Model file for the job. Use its own axes, mm. A direction names the side the tool comes from. Coordinates: 2 decimals unless noted, no trailing zeros. Loops run counter-clockwise (first coordinate to the right, second up) from the corner with the lowest first, then second, coordinate; pieces in that order, holes last. Notation, with made-up numbers: M -37.5,66 L 0.5,66 A3 ccw 0.5,71 Z; hole C 31.5,17 d7. An arc over 180 degrees is marked long. One line per question, with ' | ' between items. Start each with the question number.
```python
from build123d import *

# Parameters (mm, degrees)
SKETCH_1_W      = 190
SKETCH_1_H      = 164
EXTRUDE_2_DEPTH = 105
SKETCH_1_5_W    = 95
SKETCH_1_5_H    = 204
EXTRUDE_3_DEPTH = 105
SKETCH_2_R      = 39.7
EXTRUDE_4_DEPTH = 55
SKETCH_3_R      = 39.7
EXTRUDE_5_DEPTH = 45
EXTRUDE_START   = 55
SKETCH_4_R      = 39.7
EXTRUDE_6_DEPTH = 55
EXTRUDE_START_2 = 45
SKETCH_5_R      = 39.7
EXTRUDE_7_DEPTH = 45


with BuildPart() as part:
    # Sketch 1 → Extrude 2 (new body)
    with BuildSketch(Plane(origin=(0, 0, 0), x_dir=(1, 0, 0), z_dir=(0, 1, 0))):
        Rectangle(SKETCH_1_W, SKETCH_1_H)
    extrude(amount=EXTRUDE_2_DEPTH)

    # Sketch 1_5 → Extrude 3 (add)
    with BuildSketch(Plane(origin=(0, 0, 0), x_dir=(1, 0, 0), z_dir=(0, 1, 0))):
        with Locations((-47.5, 0)):
            Rectangle(SKETCH_1_5_W, SKETCH_1_5_H)
    extrude(amount=EXTRUDE_3_DEPTH)

    # Sketch 2 → Extrude 4 (add)
    with BuildSketch(Plane.XY.offset(102)):
        with Locations((-47.5, 52.5)):
            Circle(SKETCH_2_R)
    extrude(amount=EXTRUDE_4_DEPTH)

    # Sketch 3 → Extrude 5 (add)
    with BuildSketch(Plane.XY.offset(82)):
        with Locations(Location((47.5, 52.5, 0), (0, 0, 180))):
            Circle(SKETCH_3_R)
    extrude(amount=EXTRUDE_5_DEPTH)

    # Sketch 4 → Extrude 6 (add)
    with BuildSketch(Plane(origin=(0, 0, -102), x_dir=(-1, 0, 0), z_dir=(0, 0, -1)).offset(EXTRUDE_START)):
        with Locations(Location((47.5, 52.5, 0), (0, 0, 180))):
            Circle(SKETCH_4_R)
    extrude(amount=-EXTRUDE_6_DEPTH)

    # Sketch 5 → Extrude 7 (add)
    with BuildSketch(Plane(origin=(0, 0, -82), x_dir=(-1, 0, 0), z_dir=(0, 0, -1)).offset(EXTRUDE_START_2)):
        with Locations((-47.5, 52.5)):
            Circle(SKETCH_5_R)
    extrude(amount=-EXTRUDE_7_DEPTH)


solid = part.part
```
(1) 3-axis set-ups, long thin cutter, end or side, ignore diameter. For faces 5 (the face through (0, 52, 92)), 6 (the face through (48, 53, -127)), 7 (the face through (0, 52, -92)), 8 (the face through (29.18, 87.72, 104.18)), 9 (the face through (-80, 28, -102)): which of +Z, -Z, +X, -X, +Y, -Y reach the whole face in a straight line?
(2) Drill centre lines: line 1 (Z direction, x = -2, y = 84); line 2 (X direction, y = 61.5, z = -121); line 3 (Z direction, x = 29, y = 50.5). Where is each one in solid material? Low to high. Write a range as [from, to].
(3) Band-saw the part on A-A on y = 96.5. Write the cut outline in (x, z), then the cut area to 3 significant figures.
(4) Band-saw the part on D-D on z = 131.5. Write the cut outline in (x, y).
(5) Two-plate mould, pull along X, no slides. Class faces 1 (the face through (-95, 52, 1)), 2 (the face through (95, 52, 1)), 3 (the face through (48, 52, 127)), 4 (the face through (26.2, 86, -104.8)): pulls with the +X half, pulls with the -X half, needs draft (parallel to the pull), parting line crosses it, or undercut.
(6) Band-saw the part on C-C on x = 47.5. Write the cut outline in (y, z).
(7) Pin check, flat tips, straight feed: P1, Ø6, axis at y = 73.5, z = 94.5, coming from the +X side; P2, Ø10, axis at x = 21, y = 61.5, coming from the -Z side; P3, Ø16, axis at y = 76, z = -96, coming from the +X side. Stop position of each tip, or through.
(8) Band-saw the part on B-B on z = -86. Write the cut outline in (x, y), then the cut area to 3 significant figures.
Computed values:
1) face 5: +Z, +Y, -Y | face 6: -Z, +X, +Y, -Y | face 7: -Z, +Y, -Y | face 8: +Z | face 9: -Z
2) line 1: [-102, 102] | line 2: [-86.17, -8.83], [8.83, 86.17] | line 3: [-127, 127]
3) outline: M -95,-102 L 0,-102 L 0,-82 L 95,-82 L 95,82 L 0,82 L 0,102 L -95,102 Z | area: 35,000 mm^2
4) outline: C -47.5,52.5 d79.4
5) face 1: pulls with the -X half | face 2: pulls with the +X half | face 3: needs draft | face 4: undercut
6) outline: M 0,-82 L 12.8,-82 L 12.8,-127 L 92.2,-127 L 92.2,-82 L 105,-82 L 105,82 L 92.2,82 L 92.2,127 L 12.8,127 L 12.8,82 L 0,82 Z
7) P1: x = 82.88 | P2: z = -127 | P3: x = 84.05
8) outline: M -95,0 L 0,0 L 0,105 L -95,105 Z; C 47.5,52.5 d79.4 | area: 14,900 mm^2
